Geometry check sheet. Reference: drawing and pictorial views, mm from the part's lowest x, y, z. Round coordinates to 2 decimals unless told otherwise and drop trailing zeros. Loops run counter-clockwise (first coordinate to the right, second up) from the corner with the lowest first, then second, coordinate; pieces in that order, holes last. Notation, with made-up numbers: M 65.25,65 L 111.25,65 A21 ccw 111.25,99 Z; hole C 45.5,-35 d6. An arc over 180 degrees is marked long. One line per question, with ' | ' between items. Start each with the question number.
(1) Section check D-D (y = 3). Record the boundary of the cut face in (x, z) (1 decimal), and give its area (3 significant figures).
(2) Section check B-B (x = 73.5). Record the boundary of the cut face in (y, z), and give its area (3 significant figures).
(3) Thickness scan on probe 1 along Y at (x, z) = (5, 31); probe 2 along Y at (x, z) = (95, 14); probe 3 along X at (y, z) = (10, 7.5) (1 decimal). Record the ranges inside material, lowest first. Write a range as [from, to].
(4) Section check A-A (z = 20). Record the boundary of the cut face in (x, y) (1 decimal), and give its area (3 significant figures).
(5) Section check C-C (z = 30). Record the boundary of the cut face in (x, y), and give its area (3 significant figures).
(6) Draft check along X on the marked faces 1, 2 and 3. Enter one of: +X half, -X half, draft (parallel to the pull), parting line (faces both ways), or undercut.
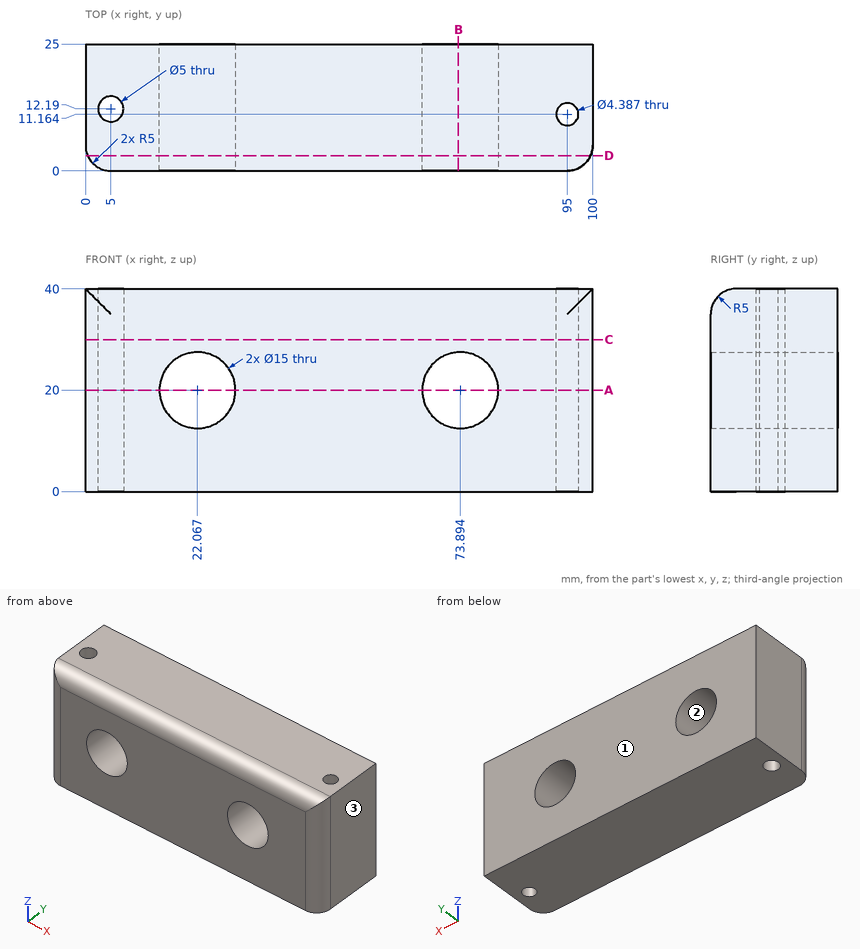
The answers:
1) outline: M 0.4,0 L 99.6,0 L 99.6,39.6 L 0.4,39.6 Z; hole C 22.1,20 d15; hole C 73.9,20 d15 | area: 3,570 mm²
2) outline: M 0,0 L 25,0 L 25,12.51 L 0,12.51 Z; M 0,27.49 L 25,27.49 L 25,40 L 5,40 A5 ccw 0,35 Z | area: 620 mm²
3) probe 1: [0, 9.69], [14.69, 25] | probe 2: [0, 8.97], [13.36, 25] | probe 3: [0, 3.8], [6.2, 93.1], [96.9, 100]
4) outline: M 0,5 A5 ccw 5,0 L 14.6,0 L 14.6,25 L 0,25 Z; M 29.6,0 L 66.4,0 L 66.4,25 L 29.6,25 Z; M 81.4,0 L 95,0 A5 ccw 100,5 L 100,25 L 81.4,25 Z; hole C 5,12.2 d5; hole C 95,11.2 d4.4 | area: 1,700 mm²
5) outline: M 0,5 A5 ccw 5,0 L 95,0 A5 ccw 100,5 L 100,25 L 0,25 Z; hole C 5,12.19 d5; hole C 95,11.16 d4.39 | area: 2,450 mm²
6) face 1: draft | face 2: undercut | face 3: +X half
